Verification items for the finished model (mm, model axes). Face numbers are marked on the shaded views. A direction names the side the tool comes from. Coordinates: 2 decimals unless noted, no trailing zeros. Order: outer loops, then holes, each group sorted by start corner. A loop starts at its lowest first (then second) coordinate and runs counter-clockwise, first axis right, second up. Notation, with made-up numbers: M 19,5.5 L 76,5.5 A23 ccw 76,40.5 Z; hole C 21.25,14 d9. An arc over 180 degrees is marked long. Use one line per item in the form item = value. Start each with the question number.
```python
from build123d import *

# Parameters (mm, degrees)
BASPROSKE_W        = 3.175
BASPROSKE_H        = 12.7
TOOTHCUT_DEPTH     = 19.238986403
TEETHCUTS_COUNT    = 22
TEETHCUTS_ANGLE    = 343.636363636
CUT_EXTRUDE1_REACH = 20.182


with BuildPart() as part:
    # BasProSke → Base-Revolve (revolve)
    with BuildSketch(Plane(origin=(0, 0, 0), x_dir=(1, 0, 0), z_dir=(0, 1, 0)), mode=Mode.PRIVATE) as base_revolve_sk:
        with Locations((1.5875, 6.35)):
            Rectangle(BASPROSKE_W, BASPROSKE_H)
    revolve(base_revolve_sk.sketch.rotate(Axis((-10, 0, 0), (1, 0, 0)), 180), axis=Axis((-10, 0, 0), (1, 0, 0)))

    # TooCutSke → ToothCut (cut, through all)
    with BuildSketch(Plane(origin=(0, 0, 0), x_dir=(0, 0, -1), z_dir=(1, 0, 0))):
        with BuildLine():
            ThreePointArc((0.618908626, 10.302292991), (0, 10.320866667), (-0.618908626, 10.302292991))
            ThreePointArc((-0.618908626, 10.302292991), (-0.876745986, 11.528868728), (-1.452383887, 12.64224609))
            ThreePointArc((-1.452383887, 12.64224609), (0, 12.7254), (1.452383887, 12.64224609))
            ThreePointArc((1.452383887, 12.64224609), (0.876745986, 11.528868728), (0.618908626, 10.302292991))
        make_face()
    toothcut = extrude(amount=TOOTHCUT_DEPTH, mode=Mode.SUBTRACT)

    # TeethCuts: ToothCut ×22 about axis
    teethcuts_axis = Axis((-10, 0, 0), (1, 0, 0))
    for i in range(1, TEETHCUTS_COUNT):
        add(toothcut.rotate(teethcuts_axis, i * TEETHCUTS_ANGLE / (TEETHCUTS_COUNT - 1)), mode=Mode.SUBTRACT)

    # Sketch1 → Cut-Extrude1 (cut, up to next)
    with BuildSketch(Plane(origin=(3.175, 0, 0), x_dir=(0, 0, -1), z_dir=(1, 0, 0)), mode=Mode.PRIVATE) as cut_extrude1_sk1:
        with BuildLine():
            Line((-1.8, -2.4), (1.8, -2.4))
            ThreePointArc((1.8, -2.4), (0, 3), (-1.8, -2.4))
        make_face()
    cut_extrude1_tool1 = extrude(cut_extrude1_sk1.sketch, amount=-CUT_EXTRUDE1_REACH, mode=Mode.PRIVATE) & part.part
    add(cut_extrude1_tool1.solids().sort_by_distance((3.175, 0.145059, 0))[0], mode=Mode.SUBTRACT)


solid = part.part
```
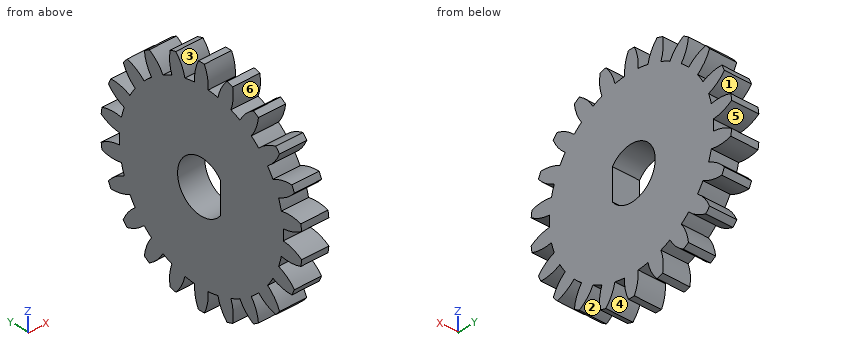
1. Tool access check on the marked faces 4, 5 and 6. Record the directions out of +Z, -Z, +X, -X, +Y, -Y that give a thin tool (end or side, any length) a straight path to the whole face; none if there is none.
2. Release check for a two-part mould opening along Z. For the marked faces 1, 2 and 3 record: pulls with the +Z half, pulls with the -Z half, needs draft (parallel to the pull), parting line crosses it, or undercut.
3. Cross-section at B-B on z = 0. Enter the section's corners in (x, y) (3 decimals), and give its area (3 significant figures).
4. Cross-section at A-A on y = 0. Enter the section's corners in (x, z) (3 decimals).
5. Depth check by flat-ended pin: P1, Ø1.5, axis at x = 1, z = -1, coming from the +Y side; P2, Ø1.6, axis at x = 2, z = 0.5, coming from the +Y side. Enter the tip coordinate at first touch or a pass-through.
6. Material ranges on line 1 along Y through (x, z) = (2.3, 0); line 2 along Z through (x, y) = (1.25, 0); line 3 along Z through (x, y) = (0.4, -11), recorded low to high.
Final values:
q1.face_4 = -Z, +X, -X
q1.face_5 = +X, -X, +Y
q1.face_6 = +X, -X
q2.face_1 = undercut
q2.face_2 = pulls with the -Z half
q2.face_3 = pulls with the +Z half
q3.outline = M 0,-10.321 L 3.175,-10.321 L 3.175,-2.4 L 0,-2.4 Z; M 0,3 L 3.175,3 L 3.175,10.321 L 0,10.321 Z
q3.area = 48.4 mm2
q4.outline = M 0,-12.7 L 3.175,-12.7 L 3.175,-3 L 0,-3 Z; M 0,3 L 3.175,3 L 3.175,12.7 L 0,12.7 Z
q5.P1 = 12.62
q5.P2 = 12.41
q6.line_1 = -10.32 to -2.4, 3 to 10.32
q6.line_2 = -12.7 to -3, 3 to 12.7
q6.line_3 = -5.61 to -4.23, -2.41 to -0.72, 0.72 to 2.41, 4.23 to 5.61
